Verification items for the finished model (mm, model axes). A direction names the side the tool comes from. Coordinates: 2 decimals unless noted, no trailing zeros. Write each loop counter-clockwise with the first axis right and the second up, starting at its lowest first coordinate (ties: lowest second). Pieces come first, ordered by that corner, then holes. Notation, with made-up numbers: (40, -16) -> (68, -16) arc R10 cw to (68, 2) -> close; hole circle Ø5 at (41.5, 53). An arc over 180 degrees is marked (long way). Answer in a Markdown table with one row per item.
```python
from build123d import *

# Parameters (mm, degrees)
F0_R      = 63.5
F1_DEPTH  = 15.875
F3_DEPTH  = 25.4
F6_R      = 6.35
F7_DEPTH  = 25.4
F8_R      = 20.32
F9_DEPTH  = 27.94
F11_R     = 20.32
F12_DEPTH = 27.686


with BuildPart() as f1:
    # F0 (on Top) → F1 (new body)
    with BuildSketch(Plane.XY):
        Circle(F0_R)
    extrude(amount=F1_DEPTH)

    # F2 (on face) → F3 (cut)
    with BuildSketch(Plane.XY.offset(15.875)):
        with BuildLine():
            Line((38.1, -50.8), (-38.1, -50.8))
            ThreePointArc((-38.1, -50.8), (0, -63.5), (38.1, -50.8))
        make_face()
    extrude(amount=-F3_DEPTH, mode=Mode.SUBTRACT)


with BuildPart() as f4_1:
    # F4: copy of F1
    add(f1.part)


with BuildPart() as f5_1:
    # F5: copy of F1
    add(f1.part)


with BuildPart() as f7_tool:
    # F6 (on face) → F7 (new body)
    with BuildSketch(Plane.XY.offset(15.875)):
        with Locations((44.45, 0)):
            Circle(F6_R)
        with Locations((0, 44.45)):
            Circle(F6_R)
        with Locations((-44.45, 0)):
            Circle(F6_R)
    extrude(amount=-F7_DEPTH)


with BuildPart() as f1_1:
    add(f1.part)

    # F7: cut by f7_tool
    add(f7_tool.part, mode=Mode.SUBTRACT)

    # F11 (on face) → F12 (join)
    with BuildSketch(Plane.XY.offset(15.875)):
        Circle(F11_R)
    extrude(amount=F12_DEPTH)


with BuildPart() as f4_1_1:
    add(f4_1.part)

    # F7: cut by f7_tool
    add(f7_tool.part, mode=Mode.SUBTRACT)


with BuildPart() as f5_1_1:
    add(f5_1.part)

    # F7: cut by f7_tool
    add(f7_tool.part, mode=Mode.SUBTRACT)


with BuildPart() as f9:
    # F8 (on face) → F9 (new body)
    with BuildSketch(Plane.XY.offset(15.875)):
        with Locations((0, 3.125413)):
            Circle(F8_R)
    extrude(amount=F9_DEPTH)


solid = f1_1.part
```
1. Section check B-B, the plane y = 0. Record the boundary of the cut face in (x, z) (3 decimals), plus the area to 3 significant figures.
Geometry says:
| item | result |
|---|---|
| outline | (-63.5, 0) -> (-50.8, 0) -> (-50.8, 15.875) -> (-63.5, 15.875) -> close; (-38.1, 0) -> (38.1, 0) -> (38.1, 15.875) -> (20.32, 15.875) -> (20.32, 43.561) -> (-20.32, 43.561) -> (-20.32, 15.875) -> (-38.1, 15.875) -> close; (50.8, 0) -> (63.5, 0) -> (63.5, 15.875) -> (50.8, 15.875) -> close |
| area | 2,740 mm^2 |
2. Section check D-D, the plane z = 9. Record the boundary of the cut face in (x, y).
Geometry says:
| item | result |
|---|---|
| outline | (-38.1, -50.8) -> (38.1, -50.8) arc R63.5 ccw (long way) to start; hole circle Ø12.7 at (-44.45, 0); hole circle Ø12.7 at (0, 44.45); hole circle Ø12.7 at (44.45, 0) |
3. Depth check by flat-ended pin: P1, Ø4, axis at x = -38.5, y = 36, coming from the +Z side (3 decimals); P2, Ø6, axis at y = 9.5, z = 16.5, coming from the +X side; P3, Ø5, axis at x = 4.5, z = 33, coming from the +Y side. Enter the tip coordinate at first touch or a pass-through.
Geometry says:
| item | result |
|---|---|
| P1 | z = 15.875 |
| P2 | x = 63.16 |
| P3 | y = 20.22 |
4. Section check A-A, the plane x = 0. Record the boundary of the cut face in (y, z) (3 decimals), plus the area to 3 significant figures.
Geometry says:
| item | result |
|---|---|
| outline | (-50.8, 0) -> (38.1, 0) -> (38.1, 15.875) -> (20.32, 15.875) -> (20.32, 43.561) -> (-20.32, 43.561) -> (-20.32, 15.875) -> (-50.8, 15.875) -> close; (50.8, 0) -> (63.5, 0) -> (63.5, 15.875) -> (50.8, 15.875) -> close |
| area | 2,740 mm^2 |
5. Section check C-C, the plane y = 44.45. Record the boundary of the cut face in (x, z) (3 decimals).
Geometry says:
| item | result |
|---|---|
| outline | (-45.348, 0) -> (-6.35, 0) -> (-6.35, 15.875) -> (-45.348, 15.875) -> close; (6.35, 0) -> (45.348, 0) -> (45.348, 15.875) -> (6.35, 15.875) -> close |
6. Thickness scan on line 1 (Y direction, x = 0, z = 9); line 2 (Z direction, x = -27.5, y = -20) (3 decimals); line 3 (X direction, y = -1, z = 26.5). Record the ranges inside material, lowest first. Write a range as from..to.
Geometry says:
| item | result |
|---|---|
| line 1 | -50.8..38.1, 50.8..63.5 |
| line 2 | 0..15.875 |
| line 3 | -20.3..20.3 |
7. Tool access check on faces 4 (the cylindrical face through (-2.645, 20.147, 29.524)), 5 (the flat face through (-1, 7, 0)). Record the directions out of +Z, -Z, +X, -X, +Y, -Y that give a thin tool (end or side, any length) a straight path to the whole face; none if there is none.
Geometry says:
| item | result |
|---|---|
| face 4 | +Z |
| face 5 | -Z, +X, -X, +Y, -Y |
8. Mould release check, pull along Y, two halves, no side actions. Record for faces 1 (the cylindrical face through (-0.827, 50.746, 8.049)), 2 (the flat face through (13, 20, 15.875)), 3 (the flat face through (1, -50.8, 8)): released by +Y, released by -Y, zero draft, split by the parting line, or undercut.
Geometry says:
| item | result |
|---|---|
| face 1 | undercut |
| face 2 | zero draft |
| face 3 | released by -Y |
